Source: CAD feature listing. Evaluate the final solid. Frame: model axes, mm. A direction names the side the tool comes from. Coordinates: 2 decimals unless noted, no trailing zeros. Order: outer loops, then holes, each group sorted by start corner. A loop starts at its lowest first (then second) coordinate and runs counter-clockwise, first axis right, second up. Notation, with made-up numbers: (82.25, -5) - (132.25, -5) arc R24 cw to (132.25, 15) - close; hole circle Ø4 at (-1.75, -21.5). An arc over 180 degrees is marked (long way). One line per question, with ' | ' between items.
from build123d import *

# Parameters (mm, degrees)
BOSS_EXTRUDE1_DEPTH  = 10
SKETCH2_W            = 6
SKETCH2_H            = 6
SKETCH2_R            = 2
BOSS_EXTRUDE2_DEPTH  = 5
SKETCH2_2_R          = 2
CUT_EXTRUDE1_DEPTH   = 11
LPATTERN2_COUNT      = 2
LPATTERN2_PITCH      = 74
LPATTERN2_COUNT_DIR2 = 2
LPATTERN2_PITCH_DIR2 = 30


with BuildPart() as part:
    # Sketch1 → Boss-Extrude1 (new body)
    with BuildSketch(Plane.XY):
        Polygon((0, 36), (6, 36), (6, 30), (74, 30), (74, 36), (80, 36), (80, 0), (0, 0), align=None)
    extrude(amount=BOSS_EXTRUDE1_DEPTH)

    # Sketch2 → Boss-Extrude2 (add)
    with BuildSketch(Plane.XY.offset(10)):
        with Locations((3, 33)):
            Rectangle(SKETCH2_W, SKETCH2_H)
        with Locations((3, 33)):
            Circle(SKETCH2_R, mode=Mode.SUBTRACT)
    boss_extrude2 = extrude(amount=BOSS_EXTRUDE2_DEPTH)

    # Sketch2<2> → Cut-Extrude1 (cut, through all)
    with BuildSketch(Plane.XY.offset(10)):
        with Locations((3, 33)):
            Circle(SKETCH2_2_R)
    cut_extrude1 = extrude(amount=-CUT_EXTRUDE1_DEPTH, mode=Mode.SUBTRACT)

    # LPattern2: Boss-Extrude2, Cut-Extrude1 2 × 2
    with Locations(*[(i * LPATTERN2_PITCH, -j * LPATTERN2_PITCH_DIR2, 0) for i in range(LPATTERN2_COUNT) for j in range(LPATTERN2_COUNT_DIR2) if (i, j) != (0, 0)]):
        add(boss_extrude2)
        add(cut_extrude1, mode=Mode.SUBTRACT)


solid = part.part
(1) Cut plane B-B (x = 3). Return the cut outline in (y, z).
Taken from the geometry:
outline: (0, 0) - (1, 0) - (1, 15) - (0, 15) - close; (5, 0) - (31, 0) - (31, 15) - (30, 15) - (30, 10) - (6, 10) - (6, 15) - (5, 15) - close; (35, 0) - (36, 0) - (36, 15) - (35, 15) - close
(2) Cut plane A-A (y = 3). Return the cut outline in (x, z).
Taken from the geometry:
outline: (0, 0) - (1, 0) - (1, 15) - (0, 15) - close; (5, 0) - (75, 0) - (75, 15) - (74, 15) - (74, 10) - (6, 10) - (6, 15) - (5, 15) - close; (79, 0) - (80, 0) - (80, 15) - (79, 15) - close
(3) Material intervals for L1, parallel to Y at x = 77, z = 4.75; L2, parallel to Y at x = 77, z = 11.55; L3, parallel to Z at x = 6.5, y = 21.5, sorted ascending. Write a range as from..to.
Taken from the geometry:
L1: y = 0..1, 5..31, 35..36 | L2: y = 0..1, 5..6, 30..31, 35..36 | L3: z = 0..10
(4) Set-up query: faces 5 (the flat face through (6, 3, 12)), 6 (the flat face through (40, 30, 5)), 7 (the flat face through (3, 6, 12)), 8 (the flat face through (75, 34, 15)). Return all of +Z, -Z, +X, -X, +Y, -Y with unobstructed straight access to the full face (end or side cutting, diameter ignored); none if empty.
Taken from the geometry:
face 5: +Z, +Y, -Y | face 6: +Z, -Z, +Y | face 7: +Z, +X, -X | face 8: +Z, +X, -X, +Y, -Y
(5) Pull-direction query (Y, two-part tool) for faces 1 (the flat face through (0, 18, 6)), 2 (the flat face through (3, 30, 12)), 3 (the flat face through (39, 0, 6)), 4 (the flat face through (41, 15, 10)); classes: pulls with the +Y half, pulls with the -Y half, needs draft (parallel to the pull), parting line crosses it, or undercut.
Taken from the geometry:
face 1: needs draft | face 2: undercut | face 3: pulls with the -Y half | face 4: undercut
(6) Cut plane C-C (z = 6). Return the cut outline in (x, y), and give its area (3 significant figures).
Taken from the geometry:
outline: (0, 0) - (80, 0) - (80, 36) - (74, 36) - (74, 30) - (6, 30) - (6, 36) - (0, 36) - close; hole circle Ø4 at (3, 3); hole circle Ø4 at (3, 33); hole circle Ø4 at (77, 3); hole circle Ø4 at (77, 33) | area: 2,420 mm²
(7) Pin query (flat end, axial travel): P1, Ø4, axis at x = 53.5, z = 6, coming from the +Y side; P2, Ø3, axis at x = 44.5, y = 23.5, coming from the +Z side. Return the tip coordinate at first contact, or that it passes through.
Taken from the geometry:
P1: stops at y = 30 | P2: stops at z = 10
(8) Cut plane D-D (y = 33). Return the cut outline in (x, z).
Taken from the geometry:
outline: (0, 0) - (1, 0) - (1, 15) - (0, 15) - close; (5, 0) - (6, 0) - (6, 15) - (5, 15) - close; (74, 0) - (75, 0) - (75, 15) - (74, 15) - close; (79, 0) - (80, 0) - (80, 15) - (79, 15) - close
